Autodesk Inventor part; units mm, degrees
ref_plane "YZ Plane" through (0, 0, 0) normal (1, 0, 0) x (0, 1, 0)
ref_plane "XZ Plane" through (0, 0, 0) normal (0, 1, 0) x (-1, 0, 0)
ref_plane "XY Plane" through (0, 0, 0) normal (0, 0, 1) x (1, 0, 0)
sketch "Sketch1" plane through (0, 0, 0) normal (0, 0, 1) x (1, 0, 0)
  line L0 (65.5, 25) -> (-65.5, 25)
  line L1 (-65.5, 25) -> (-65.5, -25)
  line L2 (-65.5, -25) -> (65.5, -25)
  line L3 (65.5, -25) -> (65.5, 25)
  line L4 (-40.6, 25) -> (-40.6, 10)
  line L5 (-40.6, 10) -> (-50.6, 10)
  line L6 (-50.6, 10) -> (-50.6, 25)
  line L7 (-40.6, -25) -> (-40.6, -10)
  line L8 (-40.6, -10) -> (-50.6, -10)
  line L9 (-50.6, -10) -> (-50.6, -25)
  line L10 (40.6, 25) -> (40.6, 10)
  line L11 (40.6, 10) -> (50.6, 10)
  line L12 (50.6, 10) -> (50.6, 25)
  line L13 (40.6, -25) -> (40.6, -10)
  line L14 (40.6, -10) -> (50.6, -10)
  line L15 (50.6, -10) -> (50.6, -25)
  circle A0 centre (24.1, 0) radius 7.5
  circle A1 centre (-24.1, 0) radius 7.5
  circle A2 centre (24.1, 0) radius 7.5
  circle A3 centre (-24.1, 0) radius 7.5
  line L16 (0, -25) -> (0, -17)
  circle A4 centre (0, -17) radius 4.75
  dimension "d0" = 15
  dimension "d1" = 15
  dimension "d2" = 15
  dimension "d3" = 15
  dimension "d8" = 15
  dimension "d9" = 15
  dimension "d35" = 8
  dimension "d36" = 9.5
extrude "Extrusion2" add sketch "Sketch1" along normal blind 10 contours A4 | L3 L2 L15 L14 L13 L7 L8 L9 L1 L0 L6 L5 L4 L10 L11 L12
sketch "Sketch2" plane through (-40.6, 25, 0) normal (0, 1, 0) x (1, 0, 0)
  circle A0 centre (64.7, -5) radius 1.25
  circle A1 centre (16.5, -5) radius 1.25
  point P0 (40.6, 0)
  dimension "d15" = 2.5
  dimension "d16" = 2.5
extrude "Extrusion3" cut sketch "Sketch2" against normal blind 10
sketch "Sketch3" plane through (0, 0, 0) normal (0, 0, -1) x (-1, 0, 0)
  circle A0 centre (0, 0) radius 24.1
  circle A1 centre (-24.1, 0) radius 7.5
  circle A2 centre (24.1, 0) radius 7.5
  circle A3 centre (-24.1, 0) radius 5
  circle A4 centre (24.1, 0) radius 5
  dimension "d25" = 48.2
  dimension "d39" = 10
  dimension "d40" = 10
extrude "Extrusion8" cut sketch "Sketch1" along normal blind 10 contours A4
extrude "Extrusion9" add sketch "Sketch3" against normal blind 2 contours A4 A0 A2 | A0 A2 A4 | A1 A0 A3 | A0 A3 A1
fillet "Fillet1" radius 2 2 edges at (-31.6, 0, 10) (16.6, 0, 10)
properties part number "prepazka-sablona"
CAD build for the part. Positions are in the model's coordinates, mm. A direction names the side the tool comes from. Give positions to 0.01 mm unless a question says otherwise; leave off trailing zeros. Order: outer loops, then holes, each group sorted by start corner. A loop starts at its lowest first (then second) coordinate and runs counter-clockwise, first axis right, second up.
(1) Saw through at D-D, the plane x = -24.1. Give the cut face in (y, z).
(2) Tool access for faces 1 (the flat face through (24, 15, 5)), 2 (the flat face through (46, 10, 5)), 3 (the cylindrical face through (31.03, 2.87, 4.96)), 4 (the flat face through (50.6, -17, 5)): list every direction of +Z, -Z, +X, -X, +Y, -Y with a clear straight run to the whole face (end or side of a thin tool).
(3) Mould opens along X. For faces 5 (the flat face through (65.5, 0, 5)), 6 (the flat face through (58, 25, 5)), 7 (the flat face through (-50.6, -17, 5)) say: released by +X, released by -X, zero draft, split by the parting line, or undercut.
(4) Flat gauge pins, fed straight in: pin 1 (12 mm diameter, centred on x = -24.5, y = 3, fed in from +Z); pin 2 (7.5 mm diameter, centred on x = 0, y = -17, fed in from +Z); pin 3 (2 mm diameter, centred on x = 24.1, z = 5, fed in from +Y). Where does each tip first touch, or does it go through?
(5) Saw through at B-B, the plane y = -17. Give the cut face in (x, z).
(6) Saw through at C-C, the plane z = 5. State how many separate pieces and enclosed holes the cut face has, then the cut area to 3 significant figures.
(7) Saw through at A-A, the plane x = 0. Give the cut face in (y, z), then the cut area to 3 significant figures.
(8) Drill centre lines: L1, parallel to X at y = 0, z = 5.2; L2, parallel to X at y = 22.5, z = 9.5; L3, parallel to X at y = 19, z = 5. Where is each one in solid material? Low to high.
Results found:
1. outline: (-25, 0) - (-5, 0) - (-5, 2) - (-7.5, 2) - (-7.5, 8) arc R2 ccw to (-9.5, 10) - (-25, 10) - close; (5, 0) - (25, 0) - (25, 3.75) - (15, 3.75) - (15, 6.25) - (25, 6.25) - (25, 10) - (9.5, 10) arc R2 ccw to (7.5, 8) - (7.5, 2) - (5, 2) - close
2. face 1: +Y
2. face 2: +Z, -Z, +Y
2. face 3: +Z
2. face 4: +Z, -Z, -Y
3. face 5: released by +X
3. face 6: zero draft
3. face 7: undercut
4. pin 1: stops at z = 9.94
4. pin 2: passes through
4. pin 3: stops at y = 15
5. outline: (-65.5, 0) - (-50.6, 0) - (-50.6, 10) - (-65.5, 10) - close; (-40.6, 0) - (-4.75, 0) - (-4.75, 10) - (-40.6, 10) - close; (4.75, 0) - (40.6, 0) - (40.6, 10) - (4.75, 10) - close; (50.6, 0) - (65.5, 0) - (65.5, 10) - (50.6, 10) - close
6. separate pieces: 1
6. enclosed holes: 3
6. area: 5,480 mm2
7. outline: (-25, 0) - (-21.75, 0) - (-21.75, 10) - (-25, 10) - close; (-12.25, 0) - (25, 0) - (25, 10) - (-12.25, 10) - close
7. area: 405 mm2
8. L1: x = -65.5 to -31.6, -16.6 to 16.6, 31.6 to 65.5
8. L2: x = -65.5 to -50.6, -40.6 to 40.6, 50.6 to 65.5
8. L3: x = -65.5 to -50.6, -40.6 to -25.35, -22.85 to 22.85, 25.35 to 40.6, 50.6 to 65.5
